```python
from build123d import *

# Parameters (mm, degrees)
SALIENTE_EXTRUIR1_DEPTH = 3


with BuildPart() as part:
    # Croquis1 → Saliente-Extruir1 (new body)
    with BuildSketch(Plane.XY):
        Polygon((-175, -97), (-165, -97), (-165, -100), (-155, -100), (-155, -97), (-145, -97), (-145, -100), (-135, -100), (-135, -97), (-125, -97), (-125, -100), (-115, -100), (-115, -97), (-105, -97), (-105, -100), (-95, -100), (-95, -97), (-85, -97), (-85, -100), (-75, -100), (-75, -97), (-65, -97), (-65, -100), (-55, -100), (-55, -97), (-45, -97), (-45, -100), (-35, -100), (-35, -97), (-25, -97), (-25, -100), (-15, -100), (-15, -97), (-5, -97), (-5, -100), (5, -100), (5, -97), (15, -97), (15, -100), (25, -100), (25, -97), (35, -97), (35, -100), (45, -100), (45, -97), (55, -97), (55, -100), (65, -100), (65, -97), (75, -97), (75, -100), (85, -100), (85, -97), (95, -97), (95, -100), (105, -100), (105, -97), (115, -97), (115, -100), (125, -100), (125, -97), (135, -97), (135, -100), (145, -100), (145, -97), (155, -97), (155, -100), (165, -100), (165, -97), (175, -97), (175, -90), (172, -90), (172, -80), (175, -80), (175, -70), (172, -70), (172, -60), (175, -60), (175, -50), (172, -50), (172, -40), (175, -40), (175, -30), (172, -30), (172, -20), (175, -20), (175, -10), (172, -10), (172, 0), (175, 0), (175, 10), (172, 10), (172, 20), (175, 20), (175, 30), (172, 30), (172, 40), (175, 40), (175, 50), (172, 50), (172, 60), (175, 60), (175, 70), (172, 70), (172, 80), (175, 80), (175, 90), (172, 90), (172, 97), (165, 97), (165, 100), (155, 100), (155, 97), (145, 97), (145, 100), (135, 100), (135, 97), (125, 97), (125, 100), (115, 100), (115, 97), (105, 97), (105, 100), (95, 100), (95, 97), (85, 97), (85, 100), (75, 100), (75, 97), (65, 97), (65, 100), (55, 100), (55, 97), (45, 97), (45, 100), (35, 100), (35, 97), (25, 97), (25, 100), (15, 100), (15, 97), (5, 97), (5, 100), (-5, 100), (-5, 97), (-15, 97), (-15, 100), (-25, 100), (-25, 97), (-35, 97), (-35, 100), (-45, 100), (-45, 97), (-55, 97), (-55, 100), (-65, 100), (-65, 97), (-75, 97), (-75, 100), (-85, 100), (-85, 97), (-95, 97), (-95, 100), (-105, 100), (-105, 97), (-115, 97), (-115, 100), (-125, 100), (-125, 97), (-135, 97), (-135, 100), (-145, 100), (-145, 97), (-155, 97), (-155, 100), (-165, 100), (-165, 97), (-172, 97), (-172, 90), (-175, 90), (-175, 80), (-172, 80), (-172, 70), (-175, 70), (-175, 60), (-172, 60), (-172, 50), (-175, 50), (-175, 40), (-172, 40), (-172, 30), (-175, 30), (-175, 20), (-172, 20), (-172, 10), (-175, 10), (-175, 0), (-172, 0), (-172, -10), (-175, -10), (-175, -20), (-172, -20), (-172, -30), (-175, -30), (-175, -40), (-172, -40), (-172, -50), (-175, -50), (-175, -60), (-172, -60), (-172, -70), (-175, -70), (-175, -80), (-172, -80), (-172, -90), (-175, -90), align=None)
    extrude(amount=SALIENTE_EXTRUIR1_DEPTH)


solid = part.part
```
Source: CAD feature listing. Evaluate the final solid. Frame: model axes, mm. Round coordinates to 2 decimals unless told otherwise and drop trailing zeros. Loops run counter-clockwise (first coordinate to the right, second up) from the corner with the lowest first, then second, coordinate; pieces in that order, holes last.
1. Contact query for flat-ended pins moving along their axis: pin 1 (1.5 mm diameter, centred on y = 98, z = 1.5, fed in from +X); pin 2 (0.9 mm diameter, centred on x = 89.5, z = 2, fed in from -Y); pin 3 (1.5 mm diameter, centred on y = -98.5, z = 1.5, fed in from -X). Output: stop coordinate, or through.
2. Section query A-A on x = 151. Output: boundary loops of the cut face in (y, z).
3. Ray query, L1, parallel to X at y = -65, z = 1.75; L2, parallel to Y at x = 10.5, z = 1.45. Return the intervals inside material, ascending.
4. Section query B-B on y = 76. Output: boundary loops of the cut face in (x, z).
Answers below:
1. pin 1: stops at x = 165
1. pin 2: stops at y = -97
1. pin 3: stops at x = -165
2. outline: (-97, 0) - (97, 0) - (97, 3) - (-97, 3) - close
3. L1: x = -172 to 172
3. L2: y = -97 to 97
4. outline: (-172, 0) - (172, 0) - (172, 3) - (-172, 3) - close
